from build123d import *

# Parameters (mm, degrees)
SKETCH1_W           = 40.64
SKETCH1_H           = 20.32
BOSS_EXTRUDE1_DEPTH = 2
FILLET1_R           = 2.54
SKETCH3_W           = 21.9202
SKETCH3_H           = 14.2494
BOSS_EXTRUDE3_DEPTH = 2.064


with BuildPart() as part:
    # Sketch1 → Boss-Extrude1 (new body)
    with BuildSketch(Plane.XY):
        Rectangle(SKETCH1_W, SKETCH1_H)
    extrude(amount=BOSS_EXTRUDE1_DEPTH)

    # Fillet1
    fillet1_edges = [part.edges().sort_by_distance(p)[0] for p in [
        (20.32, -10.16, 1),
        (-20.32, -10.16, 1),
        (-20.32, 10.16, 1),
        (20.32, 10.16, 1),
    ]]
    fillet(fillet1_edges, radius=FILLET1_R)

    # Sketch3 → Boss-Extrude3 (add)
    with BuildSketch(Plane.XY):
        with Locations((3.1369, 0)):
            Rectangle(SKETCH3_W, SKETCH3_H)
    extrude(amount=-BOSS_EXTRUDE3_DEPTH)


solid = part.part
Build history of the part. All positions in model axes, mm. A direction names the side the tool comes from. Give positions to 0.01 mm unless a question says otherwise; leave off trailing zeros. Order: outer loops, then holes, each group sorted by start corner. A loop starts at its lowest first (then second) coordinate and runs counter-clockwise, first axis right, second up. Notation, with made-up numbers: M 5.5,24.5 L 47.5,24.5 A21 cw 47.5,55.5 Z; hole C 67,61 d1. An arc over 180 degrees is marked long. Put each result on its own line as item: value.
Item 1: 3-axis set-ups, long thin cutter, end or side, ignore diameter. For faces 1 (the flat face through (3, 0, -2.064)), 2 (the flat face through (-7.823, 0, -1)), 3 (the flat face through (14.097, 0, -1)), 4 (the flat face through (3, 7.125, -1)), 5 (the flat face through (3, -7.125, -1)): which of +Z, -Z, +X, -X, +Y, -Y reach the whole face in a straight line?
From the geometry:
face 1: -Z, +X, -X, +Y, -Y
face 2: -Z, -X, +Y, -Y
face 3: -Z, +X, +Y, -Y
face 4: -Z, +X, -X, +Y
face 5: -Z, +X, -X, -Y
Item 2: Slice it at D-D, the plane x = -10.5. Write the cut outline in (y, z), plus the area to 3 significant figures.
From the geometry:
outline: M -10.16,0 L 10.16,0 L 10.16,2 L -10.16,2 Z
area: 40.6 mm2
Item 3: Slice it at C-C, the plane z = -1.65. Write the cut outline in (x, y), plus the area to 3 significant figures.
From the geometry:
outline: M -7.82,-7.12 L 14.1,-7.12 L 14.1,7.12 L -7.82,7.12 Z
area: 312 mm2
Item 4: Slice it at B-B, the plane x = 9. Write the cut outline in (y, z), plus the area to 3 significant figures.
From the geometry:
outline: M -10.16,0 L -7.12,0 L -7.12,-2.06 L 7.12,-2.06 L 7.12,0 L 10.16,0 L 10.16,2 L -10.16,2 Z
area: 70.1 mm2
Item 5: Probe line 1 (Z direction, x = -7, y = 8.5); line 2 (X direction, y = 6.5, z = -0.9); line 3 (Y direction, x = 6, z = -1.35). List the from-to ranges inside material, lowest first. Write a range as [from, to].
From the geometry:
line 1: z = [0, 2]
line 2: x = [-7.82, 14.1]
line 3: y = [-7.12, 7.12]
Item 6: Flat gauge pins, fed straight in: pin 1 Ø1 at (y, z) = (-3, -1.5) entering from +X; pin 2 Ø0.6 at (y, z) = (0, -0.5) entering from -X; pin 3 Ø1.7 at (x, z) = (5.5, -1) entering from -Y; pin 4 Ø1 at (x, z) = (-15, -1.5) entering from +Y. Where does each tip first touch, or does it go through?
From the geometry:
pin 1: stops at x = 14.1
pin 2: stops at x = -7.82
pin 3: stops at y = -7.12
pin 4: passes through
Item 7: Slice it at A-A, the plane y = 2.75. Write the cut outline in (x, z).
From the geometry:
outline: M -20.32,0 L -7.82,0 L -7.82,-2.06 L 14.1,-2.06 L 14.1,0 L 20.32,0 L 20.32,2 L -20.32,2 Z
